Verification items for this drawing (mm, ordinates from the low corner). A direction names the side the tool comes from. Round coordinates to 2 decimals unless told otherwise and drop trailing zeros. Write each loop counter-clockwise with the first axis right and the second up, starting at its lowest first coordinate (ties: lowest second). Pieces come first, ordered by that corner, then holes. Notation, with made-up numbers: M 6,61 L 12,61 A25 ccw 12,99 Z; hole C 31.5,16.5 d11. An arc over 180 degrees is marked long. Write each question's results on one line, items separated by ' | '.
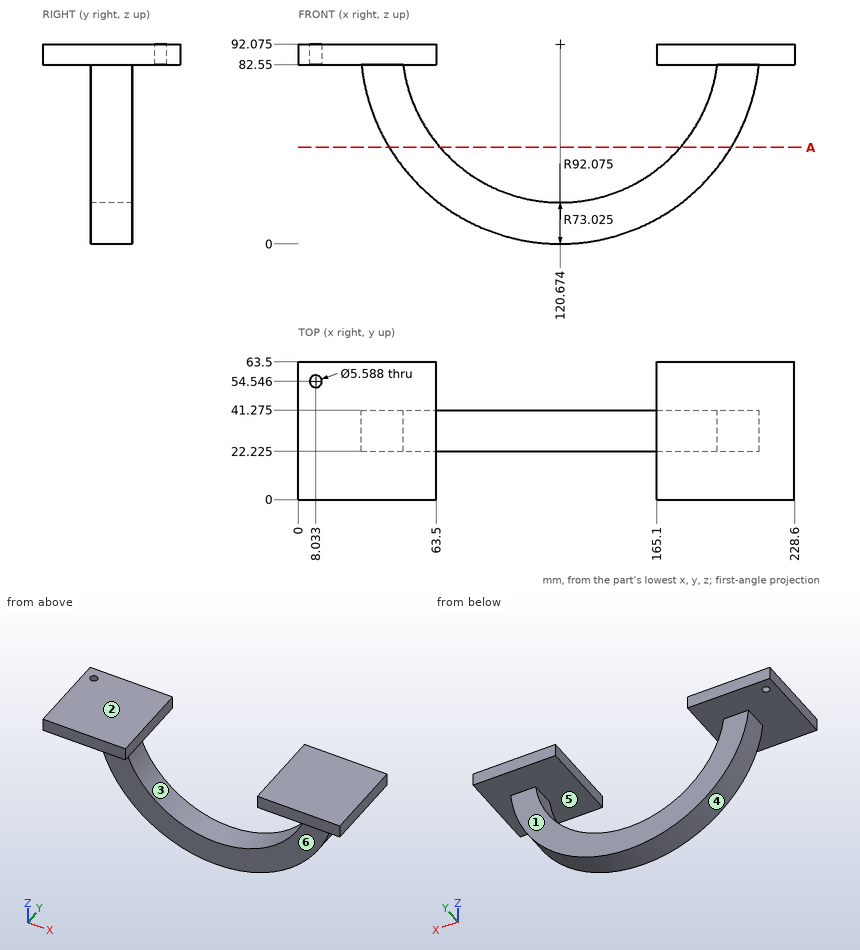
1) Sectioned sample at A-A, the plane z = 44.5. Record the cut outline in (x, y) (1 decimal), and give its area (3 significant figures).
Calculated:
outline: M 41.8,22.2 L 65.3,22.2 L 65.3,41.3 L 41.8,41.3 Z; M 176.1,22.2 L 199.5,22.2 L 199.5,41.3 L 176.1,41.3 Z | area: 893 mm²
2) Material ranges on line 1 (X direction, y = 46, z = 88); line 2 (Y direction, x = 138, z = 6) (1 decimal); line 3 (X direction, y = 24.5, z = 27) (1 decimal), recorded low to high. Write a range as [from, to].
Calculated:
line 1: x = [0, 63.5], [165.1, 228.6] | line 2: y = [22.2, 41.3] | line 3: x = [55.5, 87.5], [153.8, 185.8]
3) Draft check along X on the marked faces 3, 4, 5 and 6. Enter one of: pulls with the +X half, pulls with the -X half, needs draft (parallel to the pull), parting line crosses it, or undercut.
Calculated:
face 3: undercut | face 4: parting line crosses it | face 5: undercut | face 6: needs draft
4) Access from +Z, -Z, +X, -X, +Y, -Y to the whole of each face (thin tool, end or side, straight path). Record for the marked faces 1 and 2.
Calculated:
face 1: -Z, +X, -X, +Y | face 2: +Z, +X, -X, +Y, -Y
5) Depth check by flat-ended pin: P1, Ø5, axis at x = 35, y = 22, coming from the -Z side; P2, Ø5, axis at x = 63, y = 46.5, coming from the -Z side; P3, Ø8, axis at x = 59, y = 32.5, coming from the -Z side; P4, Ø10.5, axis at y = 23.5, z = 85, coming from the -X side. Enter the tip coordinate at first touch or a pass-through.
Calculated:
P1: stops at z = 52.6 | P2: stops at z = 82.55 | P3: stops at z = 20.3 | P4: stops at x = 0
